from build123d import *

# Parameters (mm, degrees)
CROQUIS1_W              = 920
CROQUIS1_H              = 2005
SALIENTE_EXTRUIR1_DEPTH = 1035
CROQUIS2_W              = 910
CROQUIS2_H              = 1900
CORTAR_EXTRUIR1_DEPTH   = 1025
SALIENTE_EXTRUIR2_DEPTH = 1900
SALIENTE_EXTRUIR3_DEPTH = 1900
SALIENTE_EXTRUIR4_DEPTH = 1900


with BuildPart() as part:
    # Croquis1 → Saliente-Extruir1 (new body)
    with BuildSketch(Plane.XY):
        Rectangle(CROQUIS1_W, CROQUIS1_H)
    extrude(amount=SALIENTE_EXTRUIR1_DEPTH)

    # Croquis2 → Cortar-Extruir1 (cut)
    with BuildSketch(Plane.XY.offset(1035)):
        with Locations((0, 47.5)):
            Rectangle(CROQUIS2_W, CROQUIS2_H)
    extrude(amount=-CORTAR_EXTRUIR1_DEPTH, mode=Mode.SUBTRACT)

    # Croquis3 → Saliente-Extruir2 (add)
    with BuildSketch(Plane(origin=(0, -902.5, 0), x_dir=(1, 0, 0), z_dir=(0, 1, 0))):
        Polygon((-406, -59), (-425, -59), (-425, -65), (-455, -65), (-455, -10), (-400, -10), (-400, -40), (-406, -40), align=None)
        Polygon((400, -10), (400, -40), (406, -40), (406, -59), (425, -59), (425, -65), (455, -65), (455, -10), align=None)
    extrude(amount=SALIENTE_EXTRUIR2_DEPTH)

    # Croquis4 → Saliente-Extruir3 (add)
    with BuildSketch(Plane(origin=(0, -902.5, 0), x_dir=(1, 0, 0), z_dir=(0, 1, 0))):
        Polygon((-455, -965), (-425, -965), (-425, -971), (-406, -971), (-406, -989.913190258), (-400, -989.913190258), (-400, -1019.913190258), (-455, -1019.913190258), align=None)
        Polygon((406, -971), (406, -989.913190258), (400, -989.913190258), (400, -1019.913190258), (455, -1019.913190258), (455, -965), (425, -965), (425, -971), align=None)
    extrude(amount=SALIENTE_EXTRUIR3_DEPTH)

    # Croquis5 → Saliente-Extruir4 (add)
    with BuildSketch(Plane(origin=(0, -902.5, 0), x_dir=(1, 0, 0), z_dir=(0, 1, 0))):
        Polygon((-399, -1033), (-399, -965), (-374, -965), (-374, -945), (-331, -945), (-331, -927), (-329.5, -927), (-329.5, -946.5), (-372.5, -946.5), (-372.5, -966.5), (-397.5, -966.5), (-397.5, -981.854825443), (-397.5, -1033), align=None)
        Polygon((397.5, -1033), (399, -1033), (399, -965), (374, -965), (374, -945), (331, -945), (331, -927), (329.5, -927), (329.5, -946.5), (372.5, -946.5), (372.5, -966.5), (397.5, -966.5), (397.5, -981.854825443), align=None)
    extrude(amount=SALIENTE_EXTRUIR4_DEPTH)


solid = part.part
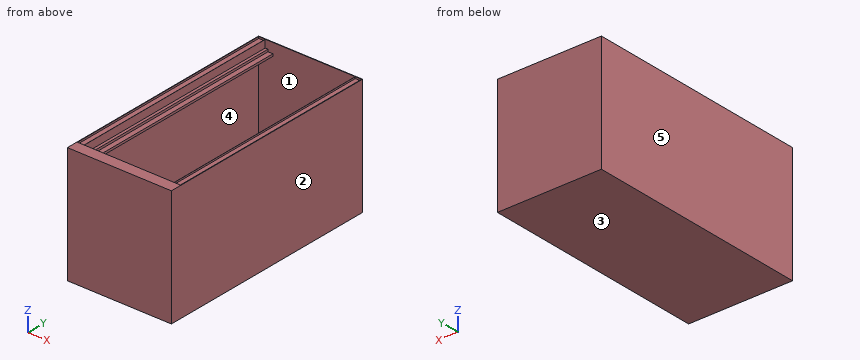
Design review of the part built by this model. Coordinates are the model's own, in mm. Face numbers are marked on the shaded views. A direction names the side the tool comes from. Round coordinates to 2 decimals unless told otherwise and drop trailing zeros. Write each loop counter-clockwise with the first axis right and the second up, starting at its lowest first coordinate (ties: lowest second). Pieces come first, ordered by that corner, then holes.
Item 1: Consider section A-A on z = 154. Give the boundary of the cut face in (x, y), and give its area (3 significant figures).
Item 2: Wall thickness on L1, parallel to X at y = 345, z = 935; L2, parallel to Z at x = -368.5, y = 426.5; L3, parallel to X at y = -680, z = 295: over which ranges is each line inside the solid? List them lowest first.
Item 3: Consider section C-C on y = 107. Count the separate pieces of the cut face and the enclosed holes in it, and give its area (3 significant figures).
Item 4: For pin 1 Ø20 at (x, y) = (383, -97.5) entering from +Z; pin 2 Ø16.5 at (x, y) = (439, -237.5) entering from +Z; pin 3 Ø10 at (x, y) = (-180, -481) entering from +Z, all flat-tipped, find the tip position at first contact; note any pin that passes through.
Item 5: Draft analysis for pull direction X (two halves, no side actions). For the marked faces 1, 2 and 3, state which applies: released by +X, released by -X, zero draft, split by the parting line, or undercut.
Item 6: Consider section B-B on x = 133.5. Give the boundary of the cut face in (y, z).
Item 7: For the marked faces 4 and 5, list the 3-axis set-ups (+Z, -Z, +X, -X, +Y, -Y) from which the entire face can be reached by the end or side of a thin tool; tool diameter is ignored.
Check values:
1. outline: (-460, -1002.5) - (460, -1002.5) - (460, 1002.5) - (-460, 1002.5) - close; hole (-455, -902.5) - (455, -902.5) - (455, 997.5) - (-455, 997.5) - close
1. area: 116,000 mm2
2. L1: x = -460 to -455, -331 to -329.5, 329.5 to 331, 455 to 460
2. L2: z = 0 to 10, 945 to 946.5
2. L3: x = -460 to -455, 455 to 460
3. separate pieces: 3
3. enclosed holes: 0
3. area: 31,000 mm2
4. pin 1: stops at z = 966.5
4. pin 2: stops at z = 1019.91
4. pin 3: stops at z = 10
5. face 1: undercut
5. face 2: released by +X
5. face 3: zero draft
6. outline: (-1002.5, 0) - (1002.5, 0) - (1002.5, 1035) - (997.5, 1035) - (997.5, 10) - (-902.5, 10) - (-902.5, 1035) - (-1002.5, 1035) - close
7. face 4: none
7. face 5: +Z, -Z, -X, +Y, -Y
